Check sheet for the modelled part. Datum: model origin and axes. Units: mm. Face numbers are marked on the shaded views. Coordinates: 2 decimals unless noted, no trailing zeros. Loops run counter-clockwise (first coordinate to the right, second up) from the corner with the lowest first, then second, coordinate; pieces in that order, holes last. Notation, with made-up numbers: (86, 30) -> (124, 30) arc R16 ccw to (124, 58) -> close; hole circle Ø5 at (4, -30). An arc over 180 degrees is marked (long way). Use one line per item in the form item = value.
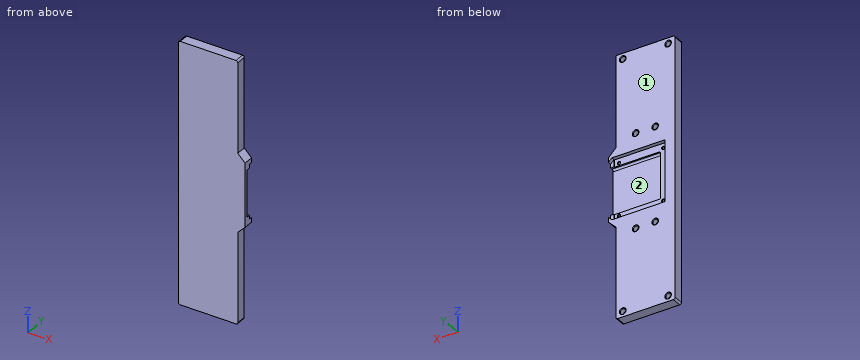
from build123d import *

# Parameters (mm, degrees)
BOSS_EXTRUDE1_DEPTH     = 11.5
SKETCH4_R               = 3.075
CUT_EXTRUDE1_DEPTH      = 6
BOSS_EXTRUDE3_DEPTH     = 11.5
CUT_EXTRUDE6_DEPTH      = 4.6
CUT_EXTRUDE3_DEPTH      = 157.057233091
CUT_EXTRUDE3_DEPTH_BACK = 3.7
SKETCH24_W              = 57
SKETCH24_H              = 54
SKETCH25_R              = 1.35
CUT_EXTRUDE4_DEPTH      = 5
CHAMFER4_SIZE           = 0.5
FILLET1_R               = 2
BOSS_EXTRUDE2_DEPTH     = 0.8
CHAMFER5_SIZE           = 0.75


with BuildPart() as part:
    # Sketch1 → Boss-Extrude1 (new body)
    with BuildSketch(Plane(origin=(0, 0, 0), x_dir=(1, 0, 0), z_dir=(0, 1, 0))):
        with BuildLine():
            Line((-34.125, 135), (-34.125, -135))
            Line((-34.125, -135), (-34.125, -148))
            ThreePointArc((-34.125, -148), (-33.539213562, -149.414213562), (-32.125, -150))
            Line((-32.125, -150), (32.125, -150))
            ThreePointArc((32.125, -150), (33.539213562, -149.414213562), (34.125, -148))
            Line((34.125, -148), (34.125, -135))
            Line((34.125, -135), (34.125, 135))
            Line((34.125, 135), (34.125, 148))
            ThreePointArc((34.125, 148), (33.539213562, 149.414213562), (32.125, 150))
            Line((32.125, 150), (-32.125, 150))
            ThreePointArc((-32.125, 150), (-33.539213562, 149.414213562), (-34.125, 148))
            Line((-34.125, 148), (-34.125, 135))
        make_face()
    extrude(amount=BOSS_EXTRUDE1_DEPTH)

    # Sketch4 → Cut-Extrude1 (cut)
    with BuildSketch(Plane(origin=(0, 11.5, 0), x_dir=(1, 0, 0), z_dir=(0, 1, 0))):
        with Locations(Location((-26.125, -143.5, 0), (0, 0, 270))):
            Circle(SKETCH4_R)
        with Locations(Location((26.125, -143.5, 0), (0, 0, 270))):
            Circle(SKETCH4_R)
        with Locations(Location((26.125, 143.5, 0), (0, 0, 270))):
            Circle(SKETCH4_R)
        with Locations(Location((-26.125, 143.5, 0), (0, 0, 270))):
            Circle(SKETCH4_R)
        with Locations(Location((-11.25, -54.175, 0), (0, 0, 270))):
            Circle(SKETCH4_R)
        with Locations(Location((11.25, -54.175, 0), (0, 0, 270))):
            Circle(SKETCH4_R)
        with Locations(Location((11.25, 54.175, 0), (0, 0, 270))):
            Circle(SKETCH4_R)
        with Locations(Location((-11.25, 54.175, 0), (0, 0, 270))):
            Circle(SKETCH4_R)
    extrude(amount=-CUT_EXTRUDE1_DEPTH, mode=Mode.SUBTRACT)

    # Sketch27 → Boss-Extrude3 (add)
    with BuildSketch(Plane(origin=(0, 11.5, 0), x_dir=(1, 0, 0), z_dir=(0, 1, 0))):
        Polygon((34.125, 45), (42.5, 36.625), (42.5, -36.625), (34.125, -45), align=None)
    extrude(amount=-BOSS_EXTRUDE3_DEPTH)

    # Sketch21 → Cut-Extrude6 (cut)
    with BuildSketch(Plane(origin=(0, 11.5, 0), x_dir=(1, 0, 0), z_dir=(0, 1, 0))):
        Polygon((42.5, 31.353553391), (42.5, -31.353553391), (38.603553391, -35.25), (-22.75, -35.25), (-22.75, 35.25), (38.603553391, 35.25), align=None)
    extrude(amount=-CUT_EXTRUDE6_DEPTH, mode=Mode.SUBTRACT)

    # Sketch24 → Cut-Extrude3 (cut, two sides: drawn at the far end of the back side and taken through both)
    with BuildSketch(Plane(origin=(0, 6.9, 0), x_dir=(1, 0, 0), z_dir=(0, 1, 0)).offset(-CUT_EXTRUDE3_DEPTH_BACK)):
        with Locations((14, 0)):
            Rectangle(SKETCH24_W, SKETCH24_H)
    extrude(amount=CUT_EXTRUDE3_DEPTH + CUT_EXTRUDE3_DEPTH_BACK, mode=Mode.SUBTRACT)

    # Sketch25 → Cut-Extrude4 (cut)
    with BuildSketch(Plane(origin=(0, 6.9, 0), x_dir=(1, 0, 0), z_dir=(0, 1, 0))):
        with Locations(Location((33.5, 30, 0), (0, 0, 270))):
            Circle(SKETCH25_R)
        with Locations(Location((-17.5, 30, 0), (0, 0, 270))):
            Circle(SKETCH25_R)
        with Locations(Location((33.5, -30, 0), (0, 0, 270))):
            Circle(SKETCH25_R)
        with Locations(Location((-17.5, -30, 0), (0, 0, 270))):
            Circle(SKETCH25_R)
    extrude(amount=-CUT_EXTRUDE4_DEPTH, mode=Mode.SUBTRACT)

    # Chamfer4
    chamfer4_edges = [part.edges().sort_by_distance(p)[0] for p in [
        (-17.5, 6.9, -31.35),
        (33.5, 6.9, 28.65),
        (-17.5, 6.9, 28.65),
        (33.5, 6.9, -31.35),
    ]]
    chamfer(chamfer4_edges, length=CHAMFER4_SIZE)

    # Fillet1
    fillet1_edges = [part.edges().sort_by_distance(p)[0] for p in [
        (14, 3.2, -27),
        (-14.5, 5.05, -27),
        (-14.5, 3.2, 0),
        (-14.5, 5.05, 27),
        (14, 3.2, 27),
    ]]
    fillet(fillet1_edges, radius=FILLET1_R)

    # Sketch26 → Boss-Extrude2 (add)
    with BuildSketch(Plane(origin=(0, 6.9, 0), x_dir=(1, 0, 0), z_dir=(0, 1, 0))):
        Polygon((38.603553391, 35.25), (38.603553391, 27), (42.5, 27), (42.5, 31.353553391), align=None)
        Polygon((42.5, -31.353553391), (38.603553391, -35.25), (38.603553391, -27), (42.5, -27), align=None)
    extrude(amount=BOSS_EXTRUDE2_DEPTH)

    # Chamfer5
    chamfer5_edges = [part.edges().sort_by_distance(p)[0] for p in [
        (26.125, 11.5, 140.425),
        (26.125, 11.5, -146.575),
        (-11.25, 11.5, 51.1),
        (11.25, 11.5, 51.1),
        (-11.25, 11.5, -57.25),
        (11.25, 11.5, -57.25),
        (-26.125, 11.5, -146.575),
        (-26.125, 11.5, 140.425),
    ]]
    chamfer(chamfer5_edges, length=CHAMFER5_SIZE)


solid = part.part
(1) Section check B-B, the plane x = -4.5. Record the boundary of the cut face in (y, z).
Established:
outline = (0, -150) -> (11.5, -150) -> (11.5, -35.25) -> (6.9, -35.25) -> (6.9, -27) -> (5.2, -27) arc R2 cw to (3.2, -25) -> (3.2, 25) arc R2 cw to (5.2, 27) -> (6.9, 27) -> (6.9, 35.25) -> (11.5, 35.25) -> (11.5, 150) -> (0, 150) -> close
(2) Scan lines: line 1 along X through (y, z) = (3, -30) (3 decimals); line 2 along Z through (x, y) = (27, 6); line 3 along Z through (x, y) = (-7, 8.25). Record each from-to range of solid material in increasing order.
Established:
line_1 = -34.125 to -18.85, -16.15 to 32.15, 34.85 to 42.5
line_2 = -150 to -146.45, -140.55 to -27, 27 to 140.55, 146.45 to 150
line_3 = -150 to -35.25, 35.25 to 150
(3) Section check C-C, the plane z = 85. Record the boundary of the cut face in (x, y) (3 decimals), plus the area to 3 significant figures.
Established:
outline = (-34.125, 0) -> (34.125, 0) -> (34.125, 11.5) -> (-34.125, 11.5) -> close
area = 785 mm²
(4) Go/stop test with flat-tipped pins: P1, Ø1.2, axis at x = 41.5, z = -30, coming from the +Y side; P2, Ø5.5, axis at x = 26.125, z = 143.5, coming from the +Y side; P3, Ø8, axis at x = 5, z = -20.5, coming from the +Y side. Record where each tip stops, or that it passes through.
Established:
P1 = 7.7
P2 = 5.5
P3 = 3.2
(5) Mould release check, pull along Z, two halves, no side actions. Record for the marked faces 1 and 2: +Z half, -Z half, draft (parallel to the pull), parting line (faces both ways), or undercut.
Established:
face_1 = draft
face_2 = undercut
(6) Section check A-A, the plane z = -143.5. Record the boundary of the cut face in (x, y) (3 decimals), plus the area to 3 significant figures.
Established:
outline = (-34.125, 0) -> (34.125, 0) -> (34.125, 11.5) -> (29.95, 11.5) -> (29.2, 10.75) -> (29.2, 5.5) -> (23.05, 5.5) -> (23.05, 10.75) -> (22.3, 11.5) -> (-22.3, 11.5) -> (-23.05, 10.75) -> (-23.05, 5.5) -> (-29.2, 5.5) -> (-29.2, 10.75) -> (-29.95, 11.5) -> (-34.125, 11.5) -> close
area = 710 mm²
